The listing builds one solid part. Answer for the finished solid, in the listing's coordinates (mm). A direction names the side the tool comes from. Coordinates: 2 decimals unless noted, no trailing zeros. Answer as CSV lines item,"result". Start each with the question number.
```python
from build123d import *

# Parameters (mm, degrees)
SKETCH2_R                = 14.463803576
BOSS_EXTRUDE1_DEPTH      = 2.5
BOSS_EXTRUDE1_TAPER      = 20
SKETCH4_W                = 8
SKETCH4_H                = 8
BOSS_EXTRUDE2_DEPTH      = 3
FILLET2_R                = 2
CIRPATTERN1_COUNT        = 4
FILLET2_OF_CIRPATTERN1_R = 2


with BuildPart() as part:
    # Sketch2 → Boss-Extrude1 (new body)
    with BuildSketch(Plane(origin=(0, 0, 0), x_dir=(1, 0, 0), z_dir=(0, 1, 0))):
        Circle(SKETCH2_R)
    extrude(amount=BOSS_EXTRUDE1_DEPTH, taper=BOSS_EXTRUDE1_TAPER)

    # Fillet1
    # an asymmetric fillet: 6, 4 mm, written as the material it takes off along each edge
    with BuildSketch(Plane(origin=(0, 2.5, 0), x_dir=(1, 0, 0), z_dir=(0, 0, -1))) as fillet1_piece_1:
        with BuildLine():
            Bezier((14.262848017, 1.94787914), (13.55387799, 0), (8.624692292, 0), weights=[1, 0.819152044, 1])
            Line((8.624692292, 0), (13.55387799, 0))
            Line((13.55387799, 0), (14.262848017, 1.94787914))
        make_face()
    revolve(axis=Axis((0, 2.5, 0), (0, -1, 0)), mode=Mode.SUBTRACT)

    # Sketch4 → Boss-Extrude2 (add)
    with BuildSketch(Plane(origin=(0, 0, 0), x_dir=(1, 0, 0), z_dir=(0, 1, 0))):
        with Locations((-12.616427752, -12.616427752)):
            Rectangle(SKETCH4_W, SKETCH4_H)
    boss_extrude2 = extrude(amount=BOSS_EXTRUDE2_DEPTH)

    # Fillet2
    fillet2_edges = [part.edges().sort_by_distance(p)[0] for p in [
        (-8.616427752, 1.5, 16.616427752),
        (-16.616427752, 1.5, 8.616427752),
        (-16.616427752, 1.5, 16.616427752),
    ]]
    fillet(fillet2_edges, radius=FILLET2_R)

    # CirPattern1: Boss-Extrude2 ×4 about axis
    cirpattern1_axis = Axis((0, 0, 0), (0, 1, 0))
    for i in range(1, CIRPATTERN1_COUNT):
        add(boss_extrude2.rotate(cirpattern1_axis, i * 360 / CIRPATTERN1_COUNT))

    # Fillet2 of CirPattern1
    fillet2_of_cirpattern1_edges = [part.edges().sort_by_distance(p)[0] for p in [
        (16.616427752, 1.5, 8.616427752),
        (8.616427752, 1.5, 16.616427752),
        (16.616427752, 1.5, 16.616427752),
        (8.616427752, 1.5, -16.616427752),
        (16.616427752, 1.5, -8.616427752),
        (16.616427752, 1.5, -16.616427752),
        (-16.616427752, 1.5, -8.616427752),
        (-8.616427752, 1.5, -16.616427752),
        (-16.616427752, 1.5, -16.616427752),
    ]]
    fillet(fillet2_of_cirpattern1_edges, radius=FILLET2_OF_CIRPATTERN1_R)


solid = part.part
```
1) Find the intervals of material crossed by line 1 (X direction, y = 2.6, z = 11.5); line 2 (Z direction, x = -12.5, y = 0.5); line 3 (Y direction, x = -1, z = 6), in increasing order. Write a range as from..to.
2) The part is cut by section A-A (x = 12). Count the separate pieces of the cut face and the enclosed holes in it, then the cut area to 3 significant figures.
3) Each of these flat-tipped pins is pushed along its axis until it touches: P1, Ø8.5, axis at x = -0.5, z = 4.5, coming from the +Y side; P2, Ø0.9, axis at y = 1, z = -10, coming from the +X side. Where does it stop, or does it pass through?
4) For a pull along Z with two mould halves and no side action, classify faces 4 (the face through (-13, 1, 16.616)), 5 (the face through (16.046, 1.521, -16.015)), 6 (the face through (13, 3, 13)), 7 (the face through (-16.05, 1.52, 9.22)) as +Z half, -Z half, draft (parallel to the pull), parting line (faces both ways), or undercut.
5) Which of the six approach directions +Z, -Z, +X, -X, +Y, -Y give full straight-line access (tool end or side, diameter ignored) to faces 1 (the face through (9.19, 1.52, 16.02)), 2 (the face through (-8.616, 2, 12)), 3 (the face through (-8.616, 2, -12))?
Completed:
1,line 1,"-16.62..-8.62, 8.62..16.62"
1,line 2,"-16.62..-8.62, -6.91..6.91, 8.62..16.62"
1,line 3,"0..2.5"
2,separate pieces,"3"
2,enclosed holes,"0"
2,area,"75.1 mm²"
3,P1,"y = 2.5"
3,P2,"x = 16.61"
4,face 4,"+Z half"
4,face 5,"-Z half"
4,face 6,"draft"
4,face 7,"undercut"
5,face 1,"+Z, +Y, -Y"
5,face 2,"+Z, +Y"
5,face 3,"-Z, +Y"
